from build123d import *

# Parameters (mm, degrees)
SKETCH1_W           = 28.2
SKETCH1_H           = 32.2
SKETCH1_R           = 1.5
BOSS_EXTRUDE1_DEPTH = 3
CHAMFER1_SIZE       = 7
CHAMFER1_SIZE2      = 4.041451884
CHAMFER3_SIZE       = 7
CHAMFER3_SIZE2      = 4.041451884
SKETCH2_W           = 28.2
SKETCH2_H           = 3
CUT_EXTRUDE1_DEPTH  = 0.5
CHAMFER4_SIZE       = 7
CHAMFER4_SIZE2      = 4.041451884
CHAMFER5_SIZE       = 7
CHAMFER5_SIZE2      = 4.041451884


with BuildPart() as part:
    # Sketch1 → Boss-Extrude1 (new body)
    with BuildSketch(Plane(origin=(0, 0, 0), x_dir=(1, 0, 0), z_dir=(0, 1, 0))):
        Rectangle(SKETCH1_W, SKETCH1_H)
        with Locations(Location((10.1, 0, 0), (0, 0, 270))):
            Circle(SKETCH1_R, mode=Mode.SUBTRACT)
        with Locations(Location((-10.1, 0, 0), (0, 0, 90))):
            Circle(SKETCH1_R, mode=Mode.SUBTRACT)
        Polygon((-6.1, -11.3), (6.1, -11.3), (6.1, 11.3), (3, 11.3), (3, 13.3), (-3, 13.3), (-3, 11.3), (-6.1, 11.3), align=None, mode=Mode.SUBTRACT)
    extrude(amount=BOSS_EXTRUDE1_DEPTH)

    # Chamfer1
    chamfer1_edges = [part.edges().sort_by_distance(p)[0] for p in [
        (14.1, 1.5, -16.1),
    ]]
    chamfer1_side = [part.faces().sort_by_distance(p)[0] for p in [
        (14.1, 1.5, 0),
    ]]
    chamfer(chamfer1_edges, length=CHAMFER1_SIZE, length2=CHAMFER1_SIZE2, reference=chamfer1_side[0])

    # Chamfer3
    chamfer3_edges = [part.edges().sort_by_distance(p)[0] for p in [
        (-14.1, 1.5, -16.1),
    ]]
    chamfer3_side = [part.faces().sort_by_distance(p)[0] for p in [
        (-14.1, 1.5, 0),
    ]]
    chamfer(chamfer3_edges, length=CHAMFER3_SIZE, length2=CHAMFER3_SIZE2, reference=chamfer3_side[0])

    # Sketch2 → Cut-Extrude1 (cut)
    with BuildSketch(Plane.XY.offset(16.1)):
        with Locations((0, 1.5)):
            Rectangle(SKETCH2_W, SKETCH2_H)
    extrude(amount=-CUT_EXTRUDE1_DEPTH, mode=Mode.SUBTRACT)

    # Chamfer4
    chamfer4_edges = [part.edges().sort_by_distance(p)[0] for p in [
        (-14.1, 1.5, 15.6),
    ]]
    chamfer4_side = [part.faces().sort_by_distance(p)[0] for p in [
        (-14.1, 1.5, 3.25),
    ]]
    chamfer(chamfer4_edges, length=CHAMFER4_SIZE, length2=CHAMFER4_SIZE2, reference=chamfer4_side[0])

    # Chamfer5
    chamfer5_edges = [part.edges().sort_by_distance(p)[0] for p in [
        (14.1, 1.5, 15.6),
    ]]
    chamfer5_side = [part.faces().sort_by_distance(p)[0] for p in [
        (14.1, 1.5, 3.25),
    ]]
    chamfer(chamfer5_edges, length=CHAMFER5_SIZE, length2=CHAMFER5_SIZE2, reference=chamfer5_side[0])


solid = part.part
Read the model definition and answer for the solid it produces. Units are mm, in the model's axes. A direction names the side the tool comes from. Round coordinates to 2 decimals unless told otherwise and drop trailing zeros. Write each loop counter-clockwise with the first axis right and the second up, starting at its lowest first coordinate (ties: lowest second). Pieces come first, ordered by that corner, then holes.
1. The part is cut by section B-B, the plane z = 0. Determine the outline of the cut face in (x, y).
2. The part is cut by section A-A, the plane x = 4.5. Determine the outline of the cut face in (y, z), then the cut area to 3 significant figures.
3. Straight lines are drawn through the part: L1, parallel to X at y = 1.2, z = 0; L2, parallel to Z at x = 0.25, y = 2.15; L3, parallel to X at y = 1.5, z = -9. For each, find the intervals that lie inside material, in ascending order.
4. Determine the mould class of faces 3 (the face through (-6.5, 0, -0.5)), 4 (the face through (-3, 1, -12)), 5 (the face through (12.05, 1.48, -12.65)) for opening direction Z: pulls with the +Z half, pulls with the -Z half, needs draft (parallel to the pull), parting line crosses it, or undercut.
5. The part is cut by section D-D, the plane z = 7.5. Determine the outline of the cut face in (x, y), then the cut area to 3 significant figures.
6. Given pin 1 Ø5 at (x, z) = (10.1, 0) entering from -Y; pin 2 Ø1 at (y, z) = (1, -12) entering from -X, each flat-ended and moving along its own axis, determine where each tip first touches the part or whether it passes through.
7. The part is cut by section C-C, the plane y = 2. Determine the outline of the cut face in (x, z).
8. Which of the six approach directions +Z, -Z, +X, -X, +Y, -Y give full straight-line access (tool end or side, diameter ignored) to faces 1 (the face through (3, 1, -12)), 2 (the face through (14.1, 1, 0))?
Values:
1. outline: (-14.1, 0) - (-11.6, 0) - (-11.6, 3) - (-14.1, 3) - close; (-8.6, 0) - (-6.1, 0) - (-6.1, 3) - (-8.6, 3) - close; (6.1, 0) - (8.6, 0) - (8.6, 3) - (6.1, 3) - close; (11.6, 0) - (14.1, 0) - (14.1, 3) - (11.6, 3) - close
2. outline: (0, -16.1) - (3, -16.1) - (3, -11.3) - (0, -11.3) - close; (0, 11.3) - (3, 11.3) - (3, 15.6) - (0, 15.6) - close
2. area: 27.3 mm2
3. L1: x = -14.1 to -11.6, -8.6 to -6.1, 6.1 to 8.6, 11.6 to 14.1
3. L2: z = -16.1 to -13.3, 11.3 to 15.6
3. L3: x = -14.1 to -6.1, 6.1 to 14.1
4. face 3: needs draft
4. face 4: undercut
4. face 5: pulls with the -Z half
5. outline: (-14.1, 0) - (-6.1, 0) - (-6.1, 3) - (-14.1, 3) - close; (6.1, 0) - (14.1, 0) - (14.1, 3) - (6.1, 3) - close
5. area: 48.0 mm2
6. pin 1: stops at y = 0
6. pin 2: stops at x = -12.71
7. outline: (-14.1, -9.1) - (-10.06, -16.1) - (10.06, -16.1) - (14.1, -9.1) - (14.1, 8.6) - (10.06, 15.6) - (-10.06, 15.6) - (-14.1, 8.6) - close; hole circle Ø3 at (-10.1, 0); hole (-6.1, -11.3) - (-3, -11.3) - (-3, -13.3) - (3, -13.3) - (3, -11.3) - (6.1, -11.3) - (6.1, 11.3) - (-6.1, 11.3) - close; hole circle Ø3 at (10.1, 0)
8. face 1: +Y, -Y
8. face 2: +Z, -Z, +X, +Y, -Y
